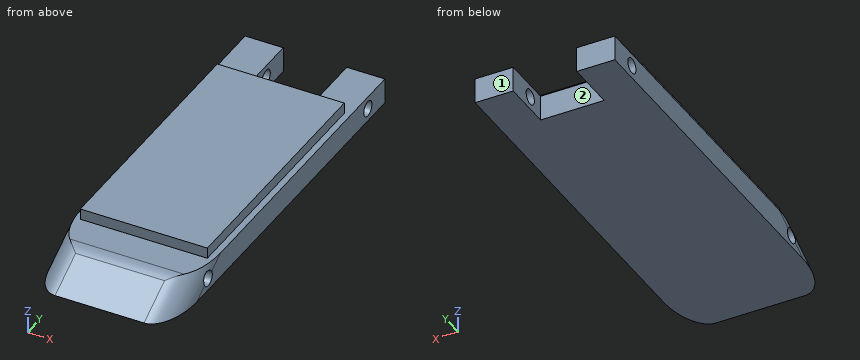
```python
from build123d import *

# Parameters (mm, degrees)
F0_W        = 180
F0_H        = 10
F1_DEPTH    = 27.5
F2_T1_DEPTH = 261.9668603717
F3_R        = 10
F4_W        = 50
F4_H        = 100
F5_DEPTH    = 4.30577
F6_W        = 25
F6_H        = 20
F7_DEPTH    = 25
F9_D        = 6
F10_D       = 6


# Not quite as in the source:
# - a fillet or chamfer that OpenCascade refuses, or shapes differently, is made with other operations: its cross-section is extruded or revolved along the edge and cut away or added


with BuildPart() as f1:
    # F0 (on Right) → F1 (new body, symmetric)
    with BuildSketch(Plane.YZ):
        with Locations((10, -5.5927829817)):
            Rectangle(F0_W, F0_H)
    extrude(amount=F1_DEPTH, both=True)

    # F2: chamfer of 40 x 23.0940107676 on 1 edges, made by hand

    # F2_s2 → F2_t1 (cut)
    with BuildSketch(Plane.YZ.offset(-130.9834301858)):
        Polygon((-40, -0.5927829817), (-80, -23.6867937493), (-80, -0.5927829817), align=None)
    extrude(amount=F2_T1_DEPTH, mode=Mode.SUBTRACT)

    # F3
    f3_edges = [f1.edges().sort_by_distance(p)[0] for p in [
        (-27.5, -48.660254, -5.592783),
        (27.5, -48.660254, -5.592783),
        (0, -40, -0.592783),
    ]]
    fillet(f3_edges, radius=F3_R)

    # F4 (on face) → F5 (join)
    with BuildSketch(Plane.XY.offset(-0.5927829817)):
        with Locations((0, 25)):
            Rectangle(F4_W, F4_H)
    extrude(amount=F5_DEPTH)

    # F6 (on face) → F7 (cut)
    with BuildSketch(Plane.XY.offset(-0.5927829817)):
        with Locations((0, 90)):
            Rectangle(F6_W, F6_H)
    extrude(amount=-F7_DEPTH, mode=Mode.SUBTRACT)

    # F9 (through all)
    with Locations(Plane.YZ.offset(27.5)):
        with Locations((-28.9948489517, -5.8634025045)):
            Hole(F9_D / 2)

    # F10 (through all)
    with Locations(Plane.YZ.offset(27.5)):
        with Locations((87.551549077, -5.5025774054)):
            Hole(F10_D / 2)


solid = f1.part
```
Can you work these out from the model? Positions are in its coordinate system, mm. Face numbers are marked on the shaded views. A direction names the side the tool comes from. Give positions to 0.01 mm unless a question says otherwise; leave off trailing zeros. Order: outer loops, then holes, each group sorted by start corner. A loop starts at its lowest first (then second) coordinate and runs counter-clockwise, first axis right, second up. Notation, with made-up numbers: M 36,39.5 L 67,39.5 A24 cw 67,50.5 Z; hole C -28.5,31.25 d4. An arc over 180 degrees is marked long. Write item = value, one per line. Start each with the question number.
Q1. Suppose I cut it at A-A (y = 42). Write out the boundary of the cut face in (x, z), plus the area to 3 significant figures.
Q2. Will these pins go through, and if not, where does the flat tip stop? pin 1 Ø3.5 at (y, z) = (87.55, -5.5) entering from +X; pin 2 Ø3.5 at (x, z) = (3, 1) entering from +Y; pin 3 Ø2 at (y, z) = (28.5, 2.5) entering from -X; pin 4 Ø5 at (y, z) = (-27.5, -1.5) entering from -X.
Q3. I need wall thicknesses on probe 1 along X at (y, z) = (83, -9); probe 2 along Y at (x, z) = (13.5, -7.25); probe 3 along Z at (x, y) = (9, 77). Which ranges of each line are inside material? Lowest first, please. Write a range as [from, to].
Q4. Suppose I cut it at C-C (x = -8). Write out the boundary of the cut face in (y, z).
Q5. For the marked faces 1 and 2, which set-ups out of +Z, -Z, +X, -X, +Y, -Y let a thin tool reach every point of the face, with its end or its side?
Q6. Suppose I cut it at D-D (y = 78). Write out the boundary of the cut face in (x, z), plus the area to 3 significant figures.
Q7. Suppose I cut it at B-B (x = -19.5). Write out the boundary of the cut face in (y, z).
Check result:
q1.outline = M -27.5,-10.59 L 27.5,-10.59 L 27.5,-0.59 L 25,-0.59 L 25,3.71 L -25,3.71 L -25,-0.59 L -27.5,-0.59 Z
q1.area = 765 mm2
q2.pin_1 = through
q2.pin_2 = 80
q2.pin_3 = -25
q2.pin_4 = -27.49
q3.probe_1 = [-27.5, -12.5], [12.5, 27.5]
q3.probe_2 = [-51.53, -31.66], [-26.33, 85.11], [89.99, 100]
q3.probe_3 = [-10.59, -0.59]
q4.outline = M -57.32,-10.59 L 80,-10.59 L 80,-0.59 L 75,-0.59 L 75,3.71 L -25,3.71 L -25,-0.59 L -37.32,-0.59 A10 ccw -42.32,-1.93 Z; hole C -28.99,-5.86 d6
q5.face_1 = +Z, -Z, +X, -X, +Y
q5.face_2 = +Z, -Z, +Y
q6.outline = M -27.5,-10.59 L 27.5,-10.59 L 27.5,-0.59 L -27.5,-0.59 Z
q6.area = 550 mm2
q7.outline = M -56.92,-10.59 L 100,-10.59 L 100,-0.59 L 75,-0.59 L 75,3.71 L -25,3.71 L -25,-0.59 L -37.32,-0.59 A10 ccw -40.49,-1.11 Z; hole C -28.99,-5.86 d6; hole C 87.55,-5.5 d6
